Work out the finished part from the listing and answer in its coordinate system (mm). Coordinates: 2 decimals unless noted, no trailing zeros. Write each loop counter-clockwise with the first axis right and the second up, starting at its lowest first coordinate (ties: lowest second). Pieces come first, ordered by that corner, then holes. Notation, with made-up numbers: (21.25, -38) - (76.25, -38) arc R11 cw to (76.25, -32) - close; hole circle Ø10 at (-33, 36). An arc over 180 degrees is marked (long way). Use a Markdown table: item, result. Add a question column.
(1) The part is cut by section B-B, the plane z = 5. Give the vertices of the cut face in (x, y), then the cut area to 3 significant figures.
(2) The part is cut by section C-C, the plane x = 27.7. Give the vertices of the cut face in (y, z), then the cut area to 3 significant figures.
(3) The part is cut by section A-A, the plane x = 6. Give the vertices of the cut face in (y, z).
(4) The part is cut by section D-D, the plane z = 8.75. Give the vertices of the cut face in (x, y).
(5) Find the intervals of material crossed by line 1 (Y direction, x = 24.5, z = 4.5); line 2 (Z direction, x = 22.5, y = 39.5), in increasing order. Write a range as from..to.
(6) Given pin 1 Ø6 at (x, z) = (9, 13) entering from +Y, flat-ended and moving along its own axis, determine where the tip first touches the part or whether it passes through.
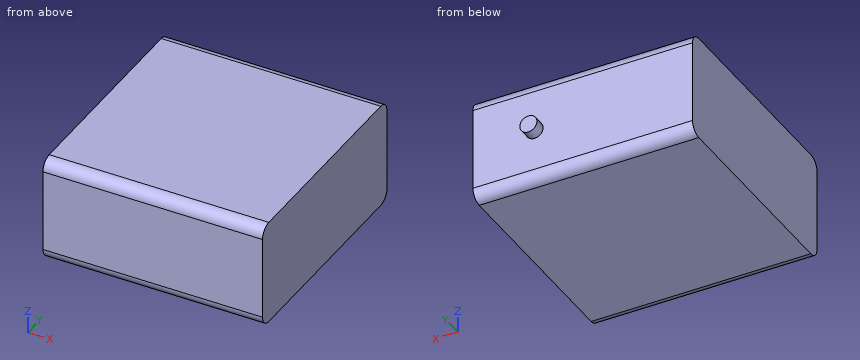
from build123d import *

# Parameters (mm, degrees)
SKETCH2_W           = 38.5
SKETCH2_H           = 40
BOSS_EXTRUDE1_DEPTH = 18.5
FILLET1_R           = 2
SKETCH3_R           = 1.5
BOSS_EXTRUDE2_DEPTH = 2


with BuildPart() as part:
    # Sketch2 → Boss-Extrude1 (new body)
    with BuildSketch(Plane.XY):
        with Locations((19.25, 20)):
            Rectangle(SKETCH2_W, SKETCH2_H)
    extrude(amount=BOSS_EXTRUDE1_DEPTH)

    # Fillet1
    fillet1_edges = [part.edges().sort_by_distance(p)[0] for p in [
        (19.25, 40, 18.5),
        (19.25, 40, 0),
        (19.25, 0, 0),
        (19.25, 0, 18.5),
    ]]
    fillet(fillet1_edges, radius=FILLET1_R)

    # Sketch3 → Boss-Extrude2 (add)
    with BuildSketch(Plane(origin=(0, 40, 0), x_dir=(1, 0, 0), z_dir=(0, 1, 0))):
        with Locations((27.7, -9.25)):
            Circle(SKETCH3_R)
    extrude(amount=BOSS_EXTRUDE2_DEPTH)


solid = part.part
Model answer:
| question | item | result |
|---|---|---|
| 1 | outline | (0, 0) - (38.5, 0) - (38.5, 40) - (0, 40) - close |
| 1 | area | 1,540 mm^2 |
| 2 | outline | (0, 2) arc R2 ccw to (2, 0) - (38, 0) arc R2 ccw to (40, 2) - (40, 7.75) - (42, 7.75) - (42, 10.75) - (40, 10.75) - (40, 16.5) arc R2 ccw to (38, 18.5) - (2, 18.5) arc R2 ccw to (0, 16.5) - close |
| 2 | area | 743 mm^2 |
| 3 | outline | (0, 2) arc R2 ccw to (2, 0) - (38, 0) arc R2 ccw to (40, 2) - (40, 16.5) arc R2 ccw to (38, 18.5) - (2, 18.5) arc R2 ccw to (0, 16.5) - close |
| 4 | outline | (0, 0) - (38.5, 0) - (38.5, 40) - (29.11, 40) - (29.11, 42) - (26.29, 42) - (26.29, 40) - (0, 40) - close |
| 5 | line 1 | 0..40 |
| 5 | line 2 | 0.68..17.82 |
| 6 | pin 1 | y = 40 |
